from build123d import *

# Parameters (mm, degrees)
SKETCH1_R           = 2.54
BOSS_EXTRUDE1_DEPTH = 3.175


with BuildPart() as part:
    # Sketch1 → Boss-Extrude1 (new body)
    with BuildSketch(Plane(origin=(0, 0, 0), x_dir=(1, 0, 0), z_dir=(0, 1, 0))):
        with BuildLine():
            ThreePointArc((-147.993238202, -11.693423436), (-142.737310664, -39.936650168), (-127.673238202, -64.398423436))
            ThreePointArc((-127.673238202, -64.398423436), (-112.609165741, -39.936650168), (-107.353238202, -11.693423436))
            ThreePointArc((-107.353238202, -11.693423436), (-51.473238202, 44.186576564), (4.406761798, -11.693423436))
            ThreePointArc((4.406761798, -11.693423436), (9.662689336, -39.936650168), (24.726761798, -64.398423436))
            ThreePointArc((24.726761798, -64.398423436), (39.790834259, -39.936650168), (45.046761798, -11.693423436))
            ThreePointArc((45.046761798, -11.693423436), (100.926761798, 44.186576564), (156.806761798, -11.693423436))
            ThreePointArc((156.806761798, -11.693423436), (162.062689336, -39.936650168), (177.126761798, -64.398423436))
            Line((177.126761798, -64.398423436), (177.126761798, 62.601576564))
            Line((177.126761798, 62.601576564), (-280.073238202, 62.601576564))
            Line((-280.073238202, 62.601576564), (-280.073238202, -64.398423436))
            ThreePointArc((-280.073238202, -64.398423436), (-265.009165741, -39.936650168), (-259.753238202, -11.693423436))
            ThreePointArc((-259.753238202, -11.693423436), (-203.873238202, 44.186576564), (-147.993238202, -11.693423436))
        make_face()
        with Locations(Location((-235.623238202, 43.551576564, 0), (0, 0, 270))):
            Circle(SKETCH1_R, mode=Mode.SUBTRACT)
        with Locations(Location((-172.123238202, 43.551576564, 0), (0, 0, 270))):
            Circle(SKETCH1_R, mode=Mode.SUBTRACT)
        with Locations(Location((-19.723238202, 43.551576564, 0), (0, 0, 270))):
            Circle(SKETCH1_R, mode=Mode.SUBTRACT)
        with Locations(Location((-83.223238202, 43.551576564, 0), (0, 0, 270))):
            Circle(SKETCH1_R, mode=Mode.SUBTRACT)
        with Locations(Location((132.676761798, 43.551576564, 0), (0, 0, 270))):
            Circle(SKETCH1_R, mode=Mode.SUBTRACT)
        with Locations(Location((69.176761798, 43.551576564, 0), (0, 0, 270))):
            Circle(SKETCH1_R, mode=Mode.SUBTRACT)
    extrude(amount=-BOSS_EXTRUDE1_DEPTH)


solid = part.part
Design review of the part built by this model. Coordinates are the model's own, in mm. A direction names the side the tool comes from. Coordinates: 2 decimals unless noted, no trailing zeros. Write each loop counter-clockwise with the first axis right and the second up, starting at its lowest first coordinate (ties: lowest second). Pieces come first, ordered by that corner, then holes. Notation, with made-up numbers: (63, 13.25) - (113, 13.25) arc R24 cw to (113, 46.25) - close; hole circle Ø9 at (5.25, -35). An arc over 180 degrees is marked (long way). One line per item, written item: value.
1) To check wall thickness, follow probe 1 along X at (y, z) = (-0.2, 18.5); probe 2 along X at (y, z) = (-2.2, 57.5); probe 3 along Z at (x, y) = (99, -2.1). State the ranges of each line that lie inside material, in increasing order.
Answer sheet:
probe 1: x = -280.07 to -260.05, -147.7 to -107.65, 4.7 to 44.75, 157.1 to 177.13
probe 2: x = -280.07 to -274.5, -133.25 to -122.1, 19.15 to 30.3, 171.55 to 177.13
probe 3: z = -62.6 to -44.15
2) Add section C-C (z = 1.5). State the section outline as (x, y) points (3 decimals), plus the area to 3 significant figures.
Answer sheet:
outline: (-280.073, -3.175) - (-258.816, -3.175) - (-258.816, 0) - (-280.073, 0) - close; (-148.931, -3.175) - (-106.416, -3.175) - (-106.416, 0) - (-148.931, 0) - close; (3.469, -3.175) - (45.984, -3.175) - (45.984, 0) - (3.469, 0) - close; (155.869, -3.175) - (177.127, -3.175) - (177.127, 0) - (155.869, 0) - close
area: 405 mm2
3) Mouldability with a two-part tool opening along X and no side actions: class faces 3 (the face through (-52.702, -1.565, -44.173)), 4 (the face through (-53, 0, -46)) as +X half, -X half, draft (parallel to the pull), parting line (faces both ways), or undercut.
Answer sheet:
face 3: undercut
face 4: draft
4) For faces 1 (the face through (-53, -3.175, -46)), 2 (the face through (39.644, -1.565, 40.314)), list the 3-axis set-ups (+Z, -Z, +X, -X, +Y, -Y) from which the entire face can be reached by the end or side of a thin tool; tool diameter is ignored.
Answer sheet:
face 1: +Z, -Z, +X, -X, -Y
face 2: +Z, +Y, -Y
5) Add section B-B (y = -0.7). State the section outline as (x, z) points.
Answer sheet:
outline: (-280.07, -62.6) - (177.13, -62.6) - (177.13, 64.4) arc R78.51 ccw to (156.81, 11.69) arc R55.88 cw to (45.05, 11.69) arc R78.51 ccw to (24.73, 64.4) arc R78.51 ccw to (4.41, 11.69) arc R55.88 cw to (-107.35, 11.69) arc R78.51 ccw to (-127.67, 64.4) arc R78.51 ccw to (-147.99, 11.69) arc R55.88 cw to (-259.75, 11.69) arc R78.51 ccw to (-280.07, 64.4) - close; hole circle Ø5.08 at (-235.62, -43.55); hole circle Ø5.08 at (-172.12, -43.55); hole circle Ø5.08 at (-83.22, -43.55); hole circle Ø5.08 at (-19.72, -43.55); hole circle Ø5.08 at (69.18, -43.55); hole circle Ø5.08 at (132.68, -43.55)
6) Add section A-A (z = 52). State the section outline as (x, y) points (3 decimals), plus the area to 3 significant figures.
Answer sheet:
outline: (-280.073, -3.175) - (-270.889, -3.175) - (-270.889, 0) - (-280.073, 0) - close; (-136.857, -3.175) - (-118.489, -3.175) - (-118.489, 0) - (-136.857, 0) - close; (15.543, -3.175) - (33.911, -3.175) - (33.911, 0) - (15.543, 0) - close; (167.943, -3.175) - (177.127, -3.175) - (177.127, 0) - (167.943, 0) - close
area: 175 mm2
7) Add section D-D (x = -54). State the section outline as (y, z) points (3 decimals), plus the area to 3 significant figures.
Answer sheet:
outline: (-3.175, -62.602) - (0, -62.602) - (0, -44.129) - (-3.175, -44.129) - close
area: 58.6 mm2
